from build123d import *

# Parameters (mm, degrees)
SKETCH_1_R          = 1.5
EXTRUDE_1_DEPTH     = 2
SKETCH_2_W          = 36.017
SKETCH_2_H          = 3
EXTRUDE_2_DEPTH     = 10
SKETCH_3_R          = 1.5
CUT_EXTRUDE_1_DEPTH = 29.168487204
FILLET_1_R          = 5


with BuildPart() as part:
    # 草图1 → 凸台-拉伸1 (new body)
    with BuildSketch(Plane.XY):
        with BuildLine():
            Line((-18.0085, 2.5), (18.0085, 2.5))
            Line((18.0085, 2.5), (18.0085, -2.5))
            Line((18.0085, -2.5), (18.0085, -12.032126861))
            ThreePointArc((18.0085, -12.032126861), (14.5085, -15.532126861), (11.0085, -12.032126861))
            Line((11.0085, -12.032126861), (11.0085, -3.595826486))
            Line((11.0085, -3.595826486), (-11.0085, -3.595826486))
            Line((-11.0085, -3.595826486), (-11.0085, -12.032126861))
            ThreePointArc((-11.0085, -12.032126861), (-14.5085, -15.532126861), (-18.0085, -12.032126861))
            Line((-18.0085, -12.032126861), (-18.0085, -2.5))
            Line((-18.0085, -2.5), (-18.0085, 2.5))
        make_face()
        with Locations((-14.5085, -12.032126861)):
            Circle(SKETCH_1_R, mode=Mode.SUBTRACT)
        with Locations(Location((14.5085, -12.032126861, 0), (0, 0, 180))):
            Circle(SKETCH_1_R, mode=Mode.SUBTRACT)
    extrude(amount=EXTRUDE_1_DEPTH)

    # 草图2 → 凸台-拉伸2 (add)
    with BuildSketch(Plane.XY.offset(2)):
        with Locations((0, 1)):
            Rectangle(SKETCH_2_W, SKETCH_2_H)
    extrude(amount=EXTRUDE_2_DEPTH)

    # 草图3 → 切除-拉伸1 (cut, through all)
    with BuildSketch(Plane(origin=(0, 2.5, 0), x_dir=(1, 0, 0), z_dir=(0, 1, 0))):
        with Locations(Location((-13.5, -7, 0), (0, 0, 180))):
            Circle(SKETCH_3_R)
        with Locations(Location((13.5, -7, 0), (0, 0, 180))):
            Circle(SKETCH_3_R)
    extrude(amount=-CUT_EXTRUDE_1_DEPTH, mode=Mode.SUBTRACT)

    # 圆角1
    fillet_1_edges = [part.edges().sort_by_distance(p)[0] for p in [
        (-18.0085, 1, 12),
        (18.0085, 1, 12),
    ]]
    fillet(fillet_1_edges, radius=FILLET_1_R)


solid = part.part
Geometry: final body of the model. Coordinates: model frame, mm. A direction names the side the tool comes from. Give positions to 0.01 mm unless a question says otherwise; leave off trailing zeros. Write each loop counter-clockwise with the first axis right and the second up, starting at its lowest first coordinate (ties: lowest second). Pieces come first, ordered by that corner, then holes.
(1) Cut plane A-A, the plane y = 0.75. Return loops of the section in (x, z).
(2) First-contact query: P1, Ø6, axis at x = 12.5, y = -8.5, coming from the +Z side; P2, Ø3.5, axis at x = 13.5, z = 7, coming from the +Y side; P3, Ø3, axis at x = 7.5, z = 4.5, coming from the -Y side; P4, Ø0.6, axis at x = 3.5, z = 0.5, coming from the -Y side. Flat tips, straight axial feed; report the tip coordinate or a pass-through.
(3) Ray query, line 1 (Y direction, x = -14, z = 8.5); line 2 (Z direction, x = -3, y = -2); line 3 (X direction, y = -10.75, z = 1.75). Return the intervals inside material, ascending.
(4) Mould query, pull axis Y, two halves, no side actions, for faces 1 (the cylindrical face through (14.59, -15.53, 0.99)), 2 (the cylindrical face through (16.007, -12.098, 0.986)), 3 (the cylindrical face through (-12.3, 1, 6.1)). Classes: released by +Y, released by -Y, zero draft, split by the parting line, or undercut.
(5) Cut plane B-B, the plane z = 8. Return loops of the section in (x, y).
(6) Cut plane D-D, the plane y = -12.75. Return loops of the section in (x, z), then the cut area to 3 significant figures.
(7) Cut plane C-C, the plane x = 12.5. Return loops of the section in (y, z), then the cut area to 3 significant figures.
(8) Access query for faces 4 (the flat face through (0, -3.596, 1)), 5 (the flat face through (0, -0.5, 7)), 6 (the flat face through (18.008, -3, 1)). Directions: +Z, -Z, +X, -X, +Y, -Y. A direction counts if a zero-diameter tool reaches every point of the face in a straight line with its end or side. Return the directions, or none.
Values follow:
1. outline: (-18.01, 0) - (18.01, 0) - (18.01, 7) arc R5 ccw to (13.01, 12) - (-13.01, 12) arc R5 ccw to (-18.01, 7) - close; hole circle Ø3 at (-13.5, 7); hole circle Ø3 at (13.5, 7)
2. P1: stops at z = 2
2. P2: stops at y = 2.5
2. P3: stops at y = -0.5
2. P4: stops at y = -3.6
3. line 1: y = -0.5 to 2.5
3. line 2: z = 0 to 2
3. line 3: x = -18.01 to -15.29, -13.73 to -11.01, 11.01 to 13.73, 15.29 to 18.01
4. face 1: released by -Y
4. face 2: undercut
4. face 3: zero draft
5. outline: (-17.91, -0.5) - (-14.62, -0.5) - (-14.62, 2.5) - (-17.91, 2.5) - close; (-12.38, -0.5) - (12.38, -0.5) - (12.38, 2.5) - (-12.38, 2.5) - close; (14.62, -0.5) - (17.91, -0.5) - (17.91, 2.5) - (14.62, 2.5) - close
6. outline: (-17.93, 0) - (-15.83, 0) - (-15.83, 2) - (-17.93, 2) - close; (-13.19, 0) - (-11.08, 0) - (-11.08, 2) - (-13.19, 2) - close; (11.08, 0) - (13.19, 0) - (13.19, 2) - (11.08, 2) - close; (15.83, 0) - (17.93, 0) - (17.93, 2) - (15.83, 2) - close
6. area: 16.9 mm2
7. outline: (-14.9, 0) - (2.5, 0) - (2.5, 5.88) - (-0.5, 5.88) - (-0.5, 2) - (-14.9, 2) - close; (-0.5, 8.12) - (2.5, 8.12) - (2.5, 12) - (-0.5, 12) - close
7. area: 58.1 mm2
8. face 4: +Z, -Z, -Y
8. face 5: +Z, +X, -X, -Y
8. face 6: +Z, -Z, +X, +Y, -Y
